Answer from the drawing. Dimensions are ordinates in mm from the lowest x, y and z of the part. A direction names the side the tool comes from. Give positions to 0.01 mm unless a question says otherwise; leave off trailing zeros. Order: outer loops, then holes, each group sorted by start corner. A loop starts at its lowest first (then second) coordinate and runs counter-clockwise, first axis right, second up. Notation, with made-up numbers: (73, -16) -> (120, -16) arc R23 cw to (120, 23) -> close; hole circle Ø5 at (19.5, 45). An arc over 180 degrees is marked (long way). Answer as CSV lines item,"result". Start each with the question number.
1) Find section A-A (y = 346). Determine the outline of the cut face in (x, z).
2) Find section C-C (y = 210.5). Determine the outline of the cut face in (x, z), and give its area (3 significant figures).
3) Flat-ended cylindrical pins translate along their axes: pin 1 Ø12.5 at (y, z) = (346, 20) entering from +X; pin 2 Ø1.5 at (x, y) = (27.5, 231) entering from -Z; pin 3 Ø22.5 at (y, z) = (46, 20) entering from +X; pin 4 Ø5.5 at (x, y) = (3, 16) entering from -Z. Find the tip coordinate at first contact, or state that the pin passes through.
4) Find section D-D (x = 16.5). Determine the outline of the cut face in (y, z), and give its area (3 significant figures).
5) Find section B-B (z = 20). Determine the outline of the cut face in (x, y), and give its area (3 significant figures).
6) Straight lines are drawn through the part: L1, parallel to Y at x = 0.8, z = 20; L2, parallel to Z at x = 13, y = 300. For each, find the intervals that lie inside material, in ascending order. Write a range as from..to.
7) For the marked faces 1 and 2, determine the directions among +Z, -Z, +X, -X, +Y, -Y from which every point of the face is accessible in a straight line to the end or side of a thin tool.
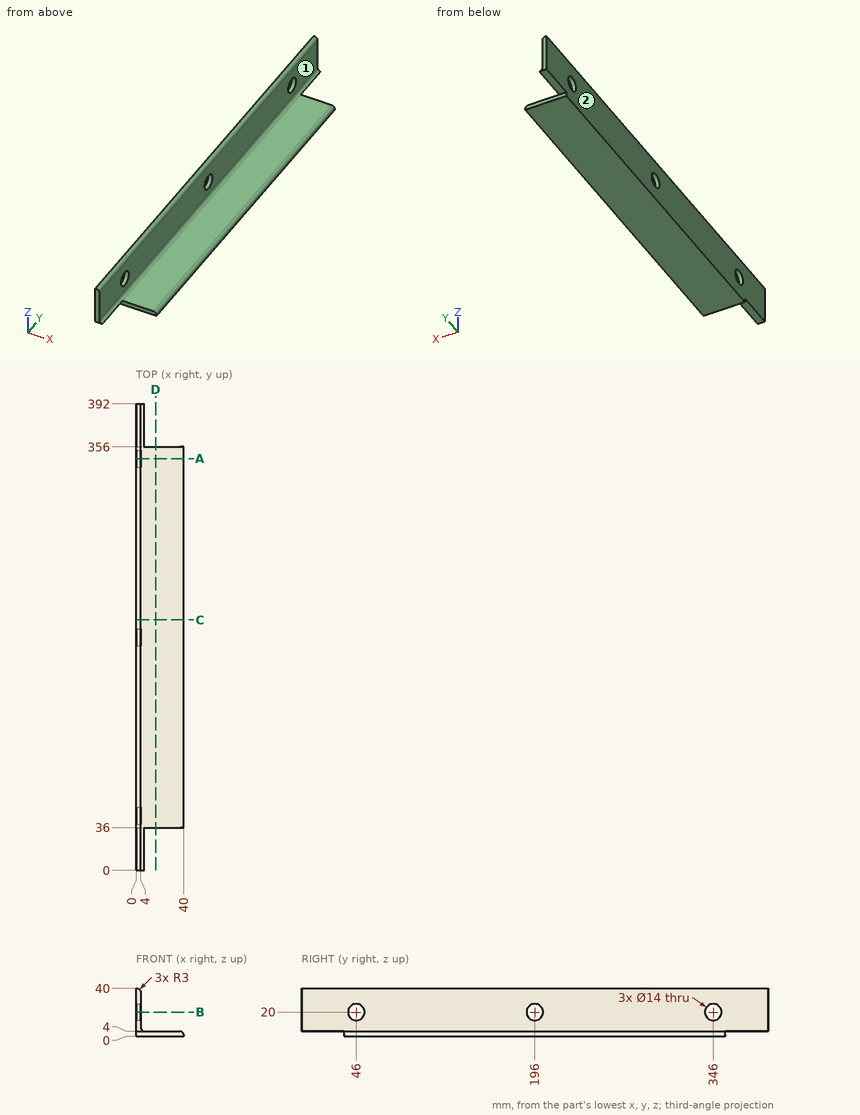
Findings below:
1,outline,"(0, 0) -> (40, 0) -> (40, 1) arc R3 ccw to (37, 4) -> (7, 4) arc R3 cw to (4, 7) -> (4, 13) -> (0, 13) -> close; (0, 27) -> (4, 27) -> (4, 37) arc R3 ccw to (1, 40) -> (0, 40) -> close"
2,outline,"(0, 0) -> (40, 0) -> (40, 1) arc R3 ccw to (37, 4) -> (7, 4) arc R3 cw to (4, 7) -> (4, 37) arc R3 ccw to (1, 40) -> (0, 40) -> close"
2,area,"302 mm²"
3,pin 1,"through"
3,pin 2,"z = 0"
3,pin 3,"x = 4"
3,pin 4,"z = 4"
4,outline,"(36, 0) -> (356, 0) -> (356, 4) -> (36, 4) -> close"
4,area,"1,280 mm²"
5,outline,"(0, 0) -> (4, 0) -> (4, 39) -> (0, 39) -> close; (0, 53) -> (4, 53) -> (4, 189) -> (0, 189) -> close; (0, 203) -> (4, 203) -> (4, 339) -> (0, 339) -> close; (0, 353) -> (4, 353) -> (4, 392) -> (0, 392) -> close"
5,area,"1,400 mm²"
6,L1,"0..39, 53..189, 203..339, 353..392"
6,L2,"0..4"
7,face 1,"+Z, +X, +Y, -Y"
7,face 2,"+Z, -Z, -X, +Y, -Y"
